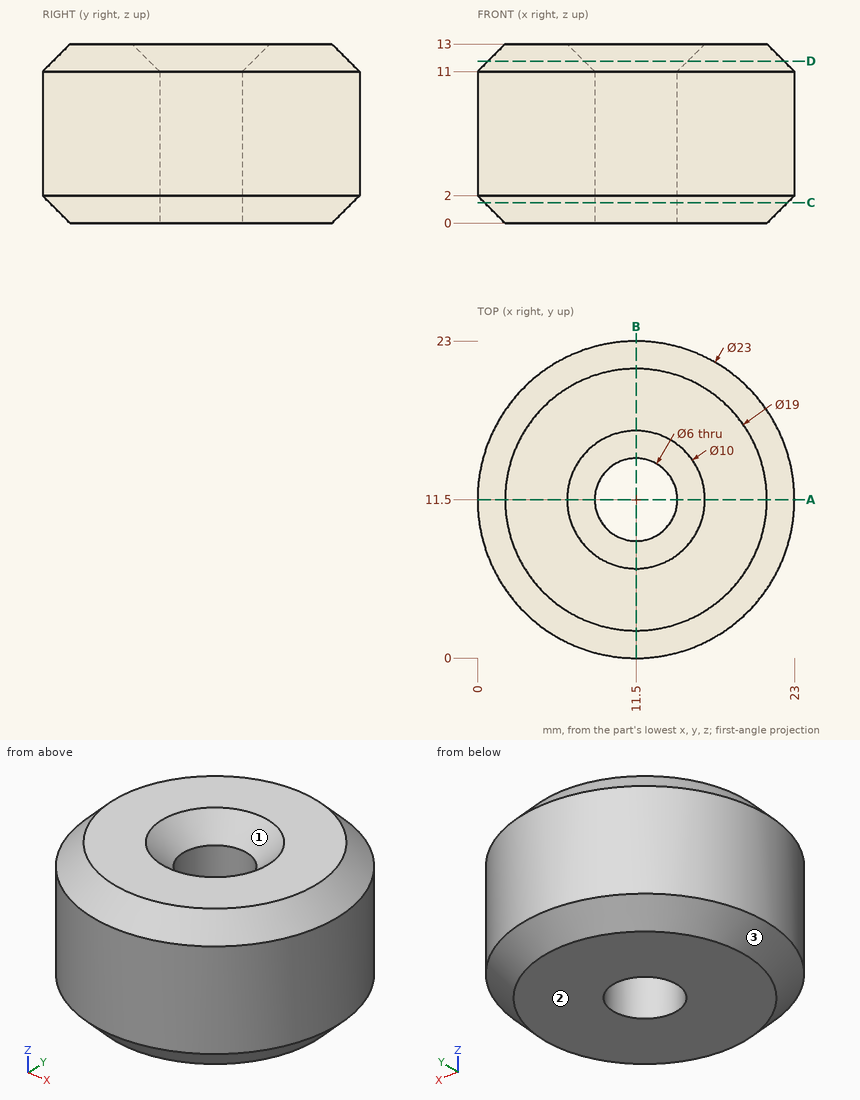
Answer from the drawing. Dimensions are ordinates in mm from the lowest x, y and z of the part. Give positions to 0.01 mm unless a question says otherwise; leave off trailing zeros. Order: outer loops, then holes, each group sorted by start corner. A loop starts at its lowest first (then second) coordinate and runs counter-clockwise, first axis right, second up. Notation, with made-up numbers: (21.5, 87.25) -> (66.5, 87.25) arc R19 cw to (66.5, 124.25) -> close; hole circle Ø11 at (-9.75, 61). An arc over 180 degrees is marked (long way). One line per item, written item: value. Start each with the question number.
(1) The part is cut by section A-A (y = 11.5). Determine the outline of the cut face in (x, z).
(2) The part is cut by section C-C (z = 1.5). Determine the outline of the cut face in (x, y).
(3) The part is cut by section D-D (z = 11.75). Determine the outline of the cut face in (x, y).
(4) Flat-ended cylindrical pins translate along their axes: P1, Ø2, axis at x = 16.5, y = 18, coming from the -Z side; P2, Ø7, axis at x = 11.5, y = 11.5, coming from the +Z side; P3, Ø5, axis at y = 17.5, z = 2, coming from the +X side; P4, Ø4, axis at y = 5, z = 7, coming from the +X side. Find the tip coordinate at first contact, or state that the pin passes through.
(5) For a pull along Y with two mould halves and no side action, classify the marked faces 1, 2 and 3 as released by +Y, released by -Y, zero draft, split by the parting line, or undercut.
(6) Straight lines are drawn through the part: L1, parallel to Y at x = 11.5, z = 3; L2, parallel to Y at x = 10.5, z = 7.25; L3, parallel to X at y = 11.25, z = 9.5. For each, find the intervals that lie inside material, in ascending order.
Taken from the geometry:
1. outline: (0, 2) -> (2, 0) -> (8.5, 0) -> (8.5, 11) -> (6.5, 13) -> (2, 13) -> (0, 11) -> close; (14.5, 0) -> (21, 0) -> (23, 2) -> (23, 11) -> (21, 13) -> (16.5, 13) -> (14.5, 11) -> close
2. outline: circle Ø22 at (11.5, 11.5); hole circle Ø6 at (11.5, 11.5)
3. outline: circle Ø21.5 at (11.5, 11.5); hole circle Ø7.5 at (11.5, 11.5)
4. P1: z = 0
4. P2: z = 11.5
4. P3: x = 22.45
4. P4: x = 22.08
5. face 1: undercut
5. face 2: zero draft
5. face 3: split by the parting line
6. L1: 0 to 8.5, 14.5 to 23
6. L2: 0.04 to 8.67, 14.33 to 22.96
6. L3: 0 to 8.51, 14.49 to 23
